Autodesk Inventor part; units mm, degrees
ref_plane "Work Plane1" through (0, -4, 9.6) normal (1, 0, 0) x (0, 0, -1)
ref_plane "YZ Plane" through (0, 0, 0) normal (1, 0, 0) x (0, 1, 0)
ref_plane "XZ Plane" through (0, 0, 0) normal (0, 1, 0) x (-1, 0, 0)
sketch "Sketch1" plane through (0, 0, 0) normal (0, 0, 1) x (1, 0, 0)
  line L0 (-4, -4) -> (4, -4)
  line L1 (4, -4) -> (4, 4)
  line L2 (4, 4) -> (-4, 4)
  line L3 (-4, 4) -> (-4, -4)
  line L4 (-4, -4) -> (4, 4) construction
  line L5 (4, -4) -> (-4, 4) construction
  circle A0 centre (0, 0) radius 2.4
  dimension "d0" = 8
  dimension "d1" = 8
  dimension "d2" = 4.8
extrude "Extrusion1" add sketch "Sketch1" along normal blind 9.6 contours L3 L2 L1 L0 | A0
extrude "Extrusion2" add sketch "Sketch1" along normal blind 11.3 contours A0
pattern_linear "Rectangular Pattern1" count 2 spacing 8 along (0, 1, 0) of "Extrusion1", "Extrusion2"
sketch "Sketch3" plane through (0, 0, 0) normal (0, 0, -1) x (-1, 0, 0)
  line L0 (4, -4) -> (-4, -4)
  line L1 (4, 12) -> (4, -4)
  line L2 (-4, 12) -> (4, 12)
  line L3 (-4, -4) -> (-4, 12)
  line L4 (2.4, 10.4) -> (2.4, -2.4)
  line L5 (2.4, -2.4) -> (-2.4, -2.4)
  line L6 (-2.4, -2.4) -> (-2.4, 10.4)
  line L7 (-2.4, 10.4) -> (2.4, 10.4)
  circle A0 centre (0, 4) radius 1.6
  line L8 (0, -2.4) -> (0, 4) construction
  point P0 (0, 0)
  dimension "d22" = 1.6
  dimension "d23" = 3.2
  dimension "d24" = 8
extrude "Extrusion6" cut sketch "Sketch3" against normal blind 8 contours L4 L5 L6 L7
sketch "Sketch2" plane through (4, -4, 9.6) normal (1, 0, 0) x (0, 0, -1)
  circle A0 centre (4, 8) radius 2.4
  circle A1 centre (4, 8) radius 3.1
  circle A2 centre (4, 8) radius 4
  line L0 (0, 0) -> (0, 16)
  line L1 (4, 4) -> (0, 4)
  line L2 (4, 12) -> (0, 12)
  line L3 (9.6, 0) -> (9.6, 16)
  line L4 (9.6, 0) -> (0, 0)
  point P0 (9.6, 4)
  dimension "d12" = 4.8
  dimension "d14" = 6.2
  dimension "d29" = 8
  dimension "d30" = 8
  dimension "d31" = 5.6
ref_plane "Work Plane1" through (0, -4, 9.6) normal (1, 0, 0) x (0, 0, -1)
extrude "Extrusion4" cut sketch "Sketch2" against normal up to surface (8 mm away) from surface at 0 contours A0
extrude "Extrusion5" cut sketch "Sketch2" against normal blind 0.8 contours A1
mirror "Mirror1" about plane through (0, -4, 9.6) normal (1, 0, 0) of "Extrusion5"
pattern_of_one "Rectangular Pattern2"
extrude "Extrusion7" add sketch "Sketch2" against normal up to surface (4.8 mm away) from surface at -1.6 contours A1 | A2 | A2 L0 L2 | L1 L0 A2
equation "\"d11\" = d0"
equation "\"d21\" = d0"
properties part number "real LEGO Technic Brick 1x2 with Holes"
Here's how the part is built. I have some questions about the finished solid (model axes, mm). A direction names the side the tool comes from. Coordinates: 2 decimals unless noted, no trailing zeros. Loops run counter-clockwise (first coordinate to the right, second up) from the corner with the lowest first, then second, coordinate; pieces in that order, holes last.
1. Imagine slicing it at C-C, the plane x = 3.5. Please give me the cut outline in (y, z), and give its area (3 significant figures).
2. Imagine slicing it at A-A, the plane y = 4. Please give me the cut outline in (x, z), and give its area (3 significant figures).
3. Imagine slicing it at B-B, the plane z = 7.25. Please give me the cut outline in (x, y), and give its area (3 significant figures).
4. I need wall thicknesses on L1, parallel to X at y = -2, z = 3.5; L2, parallel to Y at x = 0.25, z = 5.5; L3, parallel to Y at x = 3.55, z = 5.6. Which ranges of each line are inside material? Lowest first, please.
5. If we mould it in two halves opening along Y, with no side actions, what happens to faces 4 (the flat face through (0, 12, 5)), 5 (the flat face through (0, -4, 5)), 6 (the flat face through (0, 8, 11.3)), 7 (the flat face through (0, 4, 9.6))? For each: pulls with the +Y half, pulls with the -Y half, needs draft (parallel to the pull), parting line crosses it, or undercut.
6. For P1, Ø2, axis at x = 0.5, y = 4, coming from the -Z side; P2, Ø5, axis at y = 4, z = 5.6, coming from the -X side; P3, Ø0.7, axis at x = 0, y = -1.5, coming from the -Z side, each with a flat end and sliding along its axis, tell me the tip position at first contact or that it passes through.
7. Imagine slicing it at D-D, the plane y = -2. Please give me the cut outline in (x, z).
8. For faces 1 (the cylindrical face through (1.1, 2.55, 1.87)), 2 (the cylindrical face through (1.29, 5.976, 10.438)), 3 (the flat face through (-3.2, 3, 3)), which set-ups out of +Z, -Z, +X, -X, +Y, -Y let a thin tool reach every point of the face, with its end or its side?
Taken from the geometry:
1. outline: (-4, 0) - (12, 0) - (12, 9.6) - (-4, 9.6) - close; hole circle Ø6.2 at (4, 5.6)
1. area: 123 mm2
2. outline: (-4, 0) - (-2.4, 0) - (-2.4, 1.6) - (-1.6, 1.6) - (-1.6, 0) - (1.6, 0) - (1.6, 1.6) - (2.4, 1.6) - (2.4, 0) - (4, 0) - (4, 2.5) - (3.2, 2.5) - (3.2, 3.2) - (-3.2, 3.2) - (-3.2, 2.5) - (-4, 2.5) - close; (-4, 8.7) - (-3.2, 8.7) - (-3.2, 8) - (3.2, 8) - (3.2, 8.7) - (4, 8.7) - (4, 9.6) - (-4, 9.6) - close
2. area: 33.6 mm2
3. outline: (-4, -4) - (4, -4) - (4, 1.38) - (3.2, 1.38) - (3.2, 2.26) - (-3.2, 2.26) - (-3.2, 1.38) - (-4, 1.38) - close; (-4, 6.62) - (-3.2, 6.62) - (-3.2, 5.74) - (3.2, 5.74) - (3.2, 6.62) - (4, 6.62) - (4, 12) - (-4, 12) - close; hole (-2.4, -2.4) - (2.4, -2.4) - (2.4, 0) - (-2.4, 0) - close; hole (-2.4, 8) - (2.4, 8) - (2.4, 10.4) - (-2.4, 10.4) - close
3. area: 74.3 mm2
4. L1: x = -4 to -2.4, 2.4 to 4
4. L2: y = -4 to -2.4, 0 to 1.6, 6.4 to 8, 10.4 to 12
4. L3: y = -4 to 0.9, 7.1 to 12
5. face 4: pulls with the +Y half
5. face 5: pulls with the -Y half
5. face 6: needs draft
5. face 7: undercut
6. P1: stops at z = 0
6. P2: stops at x = -3.2
6. P3: stops at z = 8
7. outline: (-4, 0) - (-2.4, 0) - (-2.4, 8) - (2.4, 8) - (2.4, 0) - (4, 0) - (4, 9.6) - (1.33, 9.6) - (1.33, 11.3) - (-1.33, 11.3) - (-1.33, 9.6) - (-4, 9.6) - close
8. face 1: -Z
8. face 2: +Z
8. face 3: -X
